The model under review builds one solid part; all positions refer to its coordinate system, in mm. Round coordinates to 2 decimals unless told otherwise and drop trailing zeros. Write each loop counter-clockwise with the first axis right and the second up, starting at its lowest first coordinate (ties: lowest second). Pieces come first, ordered by that corner, then holes. Notation, with made-up numbers: (64.5, 46) -> (89.5, 46) arc R16 cw to (89.5, 55) -> close; hole circle Ø8 at (-32, -22). An arc over 180 degrees is marked (long way). Return JSON: item names as keys, results as strings. Group by question number.
1. Clearance check with flat-ended pins moving along their axes: P1, Ø8, axis at x = 388.11, z = 0.06, coming from the +Y side; P2, Ø2, axis at x = 196, z = 7.5, coming from the -Y side; P3, Ø6, axis at x = 348.5, y = -7, coming from the -Z side; P4, Ø6, axis at x = 87.5, z = -7, coming from the -Y side. State where each tip first meets the part, or that it passes through.
2. Take a section at A-A, the plane x = 366.5. Write out the cut boundary in (y, z) (3 decimals).
3. For line 1 along Z through (x, y) = (213.5, -0.5); line 2 along Y through (x, z) = (281, 5), list the stretches that pass through material, from the lowest coordinate up. Write a range as from..to.
Autodesk Inventor part; units mm, degrees
ref_plane "YZ Plane" through (0, 0, 0) normal (1, 0, 0) x (0, 1, 0)
ref_plane "XZ Plane" through (0, 0, 0) normal (0, 1, 0) x (-1, 0, 0)
ref_plane "XY Plane" through (0, 0, 0) normal (0, 0, 1) x (1, 0, 0)
sketch "Sketch1" plane through (0, 0, 0) normal (1, 0, 0) x (0, 1, 0)
  circle A0 centre (0, 0) radius 9.525
  dimension "d0" = 19.05
sketch "Sketch2" plane through (0, 0, 0) normal (0, 1, 0) x (-1, 0, 0)
  line L0 (0, 0) -> (-398.5, 0)
  dimension "d1" = 398.5
sweep "Sweep1" add profiles "Sketch1" path "Sketch2"
sketch "Sketch3" plane through (0, 0, 0) normal (0, 1, 0) x (-1, 0, 0)
  circle A0 centre (-388.1092, 0.0619) radius 5
  dimension "d4" = 10
extrude "Cut1" cut sketch "Sketch3" along normal through all both and the other way through all
sketch "Sketch4" plane through (398.5, 0, 0) normal (1, 0, 0) x (0, 0, -1)
  circle A0 centre (0, 0) radius 8.1874
extrude "Cut2" cut sketch "Sketch4" against normal through all
sketch "Sketch5" plane through (0, 0, 0) normal (0, 0, 1) x (1, 0, 0)
  circle A0 centre (13.9095, -0.404) radius 5
  dimension "d9" = 10
extrude "Cut3" cut sketch "Sketch5" along normal through all both and the other way through all
equation "\"d5\" = d4"
equation "\"d7\" = Thickness"
equation "\"d10\" = Thickness"
equation "\"BendRadius\" = Thickness"
equation "\"BendReliefWidth\" = Thickness"
equation "\"BendReliefDepth\" = 0.5 * Thickness"
equation "\"CornerReliefSize\" = 4 * Thickness"
equation "\"MinimumRemnant\" = 2 * Thickness"
equation "\"TransitionRadius\" = BendRadius"
equation "\"JacobiRadiusSize\" = BendRadius"
equation "\"GapSize\" = Thickness"
properties part number "Tubo_conexion"
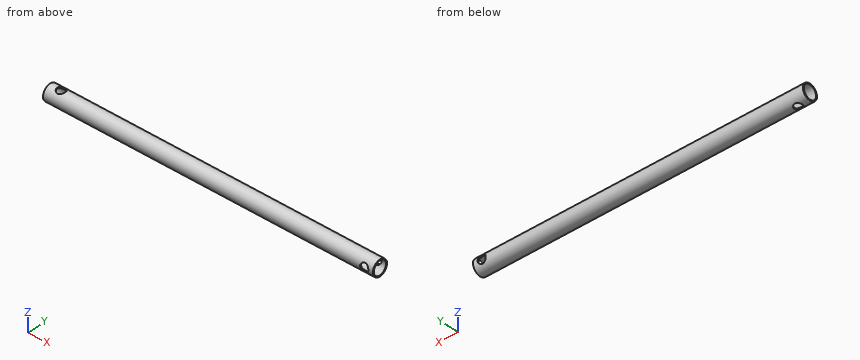
Output:
{
 "1": {"P1": "passes through", "P2": "stops at y = -6.96", "P3": "stops at z = -8.64", "P4": "stops at y = -8.64"},
 "2": {"outline": "circle Ø19.05 at (0, 0); hole circle Ø16.375 at (0, 0)"},
 "3": {"line 1": "z = -9.51..-8.17, 8.17..9.51", "line 2": "y = -8.11..-6.48, 6.48..8.11"}
}
